from build123d import *

# Parameters (mm, degrees)
PAD_DEPTH       = 24
SKETCH_R        = 4.625
SKETCH_R_2      = 3
SKETCH_W        = 8.497862
SKETCH_H        = 16.9564
POCKET_DEPTH    = 4
SKETCH003_R     = 2.6
POCKET001_DEPTH = 13
FILLET_R        = 13
FILLET001_R     = 1
SKETCH004_R     = 3.2
POCKET002_DEPTH = 3


with BuildPart() as part:
    # Sketch002 → Pad (new body, symmetric)
    with BuildSketch(Plane.YZ.offset(24)):
        Polygon((0, 4), (56.5, 4), (56.5, -8), (48.5, -8), (48.5, -4), (52.5, -4), (52.5, 0), (13, 0), (13, -13), (0, -13), (0, 0), (-68, 0), (-68, 4), align=None)
    extrude(amount=PAD_DEPTH, both=True)

    # Sketch (on Face13 of Pad) → Pocket (cut)
    with BuildSketch(Plane(origin=(24, -34, 4), x_dir=(-1, 0, 0), z_dir=(0, 0, 1))):
        with Locations((-12.025, 28)):
            Circle(SKETCH_R)
        with Locations((12.025, 28)):
            Circle(SKETCH_R)
        with Locations((12.025, -28)):
            Circle(SKETCH_R)
        with Locations((-12.025, -28)):
            Circle(SKETCH_R)
        with Locations((-12.024955, 15.059916)):
            Circle(SKETCH_R_2)
        with Locations((12.024955, 15.059916)):
            Circle(SKETCH_R_2)
        with Locations((12.024955, -15.059916)):
            Circle(SKETCH_R_2)
        with Locations((-12.024955, -15.059916)):
            Circle(SKETCH_R_2)
        with Locations((-12.001069, 0.0218)):
            Rectangle(SKETCH_W, SKETCH_H)
        with Locations((12.001069, -0.0218)):
            Rectangle(SKETCH_W, SKETCH_H)
    extrude(amount=-POCKET_DEPTH, mode=Mode.SUBTRACT)

    # Sketch003 (on Face30 of Pocket) → Pocket001 (cut)
    with BuildSketch(Plane(origin=(24, 0, 0), x_dir=(0, 0, -1), z_dir=(0, -1, 0))):
        with Locations((9.313336, 0)):
            Circle(SKETCH003_R)
    extrude(amount=-POCKET001_DEPTH, mode=Mode.SUBTRACT)

    # Fillet
    fillet_edges = [part.edges().sort_by_distance(p)[0] for p in [
        (48, 6.5, -13),
        (0, 6.5, -13),
    ]]
    fillet(fillet_edges, radius=FILLET_R)

    # Fillet001
    fillet001_edges = [part.edges().sort_by_distance(p)[0] for p in [
        (24, 56.5, 4),
        (0, 56.5, -2),
        (48, 56.5, -2),
        (24, 56.5, -8),
        (0, 52.5, -8),
        (48, 52.5, -8),
        (24, 48.5, -8),
        (0, 6.5, 0),
        (0, 32.75, 0),
        (0, -34, 0),
        (0, 52.5, -2),
        (0, -68, 2),
        (0, 50.5, -4),
        (0, -34, 4),
        (0, 48.5, -6),
        (0, 28.25, 4),
        (48, 6.5, 0),
        (48, 32.75, 0),
        (48, -34, 0),
        (48, 52.5, -2),
        (48, -68, 2),
        (48, 50.5, -4),
        (48, -34, 4),
        (48, 48.5, -6),
        (48, 28.25, 4),
        (24, -68, 4),
        (24, -68, 0),
        (24, 48.5, -4),
    ]]
    fillet(fillet001_edges, radius=FILLET001_R)

    # Sketch004 (on Face5 of Fillet001) → Pocket002 (cut)
    with BuildSketch(Plane(origin=(24, 0, 0), x_dir=(0, 0, -1), z_dir=(0, -1, 0))):
        with Locations((9.313336, 0)):
            Circle(SKETCH004_R)
    extrude(amount=-POCKET002_DEPTH, mode=Mode.SUBTRACT)


solid = part.part
Read the model definition and answer for the solid it produces. Units are mm, in the model's axes. A direction names the side the tool comes from. Coordinates: 2 decimals unless noted, no trailing zeros. Loops run counter-clockwise (first coordinate to the right, second up) from the corner with the lowest first, then second, coordinate; pieces in that order, holes last. Notation, with made-up numbers: (-28.75, -8.75) - (8.25, -8.75) arc R16 cw to (8.25, 1.25) - close; hole circle Ø8 at (-20, 42.25). An arc over 180 degrees is marked (long way). Answer in a Markdown table with one row per item.
Q1. The mould has two halves that part along Y. Classify faces 1 (the flat face through (24, 56.5, -2)), 2 (the flat face through (48, 4, 1)), 3 (the cylindrical face through (7.7, -4.23, 2.03)): pulls with the +Y half, pulls with the -Y half, needs draft (parallel to the pull), parting line crosses it, or undercut.
Here are the results:
| item | result |
|---|---|
| face 1 | pulls with the +Y half |
| face 2 | needs draft |
| face 3 | undercut |
Q2. For faces 4 (the flat face through (24, 53, -8)), 5 (the flat face through (7.75, -34, 2)), 6 (the flat face through (24, 51, -4)), determine the directions among +Z, -Z, +X, -X, +Y, -Y from which every point of the face is accessible in a straight line to the end or side of a thin tool.
Here are the results:
| item | result |
|---|---|
| face 4 | -Z, +X, -X, +Y |
| face 5 | +Z, -Z |
| face 6 | +X, -X |
Q3. Find section B-B on x = 24. Write down the section's boundary in (y, z), plus the area to 3 significant figures.
Here are the results:
| item | result |
|---|---|
| outline | (-68, 1) arc R1 ccw to (-67, 0) - (0, 0) - (0, -6.11) - (3, -6.11) - (3, -6.71) - (13, -6.71) - (13, 0) - (52.5, 0) - (52.5, -4) - (49.5, -4) arc R1 ccw to (48.5, -5) - (48.5, -7) arc R1 ccw to (49.5, -8) - (55.5, -8) arc R1 ccw to (56.5, -7) - (56.5, 3) arc R1 ccw to (55.5, 4) - (-67, 4) arc R1 ccw to (-68, 3) - close; (0, -13) - (13, -13) - (13, -11.91) - (3, -11.91) - (3, -12.51) - (0, -12.51) - close |
| area | 643 mm^2 |
Q4. Straight lines are drawn through the part: line 1 along X through (y, z) = (-6, 2.7); line 2 along Y through (x, z) = (20.5, -0.5); line 3 along Y through (x, z) = (25, -6.5). For each, find the intervals that lie inside material, in ascending order. Write a range as [from, to].
Here are the results:
| item | result |
|---|---|
| line 1 | x = [0, 7.35], [16.6, 31.4], [40.65, 48] |
| line 2 | y = [0, 13], [52.5, 56.5] |
| line 3 | y = [3, 13], [48.5, 56.5] |
Q5. Find section A-A on y = -30. Write down the section's boundary in (x, z), plus the area to 3 significant figures.
Here are the results:
| item | result |
|---|---|
| outline | (0, 1) arc R1 ccw to (1, 0) - (7.75, 0) - (7.75, 4) - (1, 4) arc R1 ccw to (0, 3) - close; (16.25, 0) - (31.75, 0) - (31.75, 4) - (16.25, 4) - close; (40.25, 0) - (47, 0) arc R1 ccw to (48, 1) - (48, 3) arc R1 ccw to (47, 4) - (40.25, 4) - close |
| area | 123 mm^2 |
Q6. Given P1, Ø10, axis at y = -15.5, z = -4.5, coming from the -X side; P2, Ø2, axis at x = 14, z = -1.5, coming from the -Y side; P3, Ø6, axis at x = 24, z = -9.31, coming from the -Y side, each flat-ended and moving along its own axis, determine where each tip first touches the part or whether it passes through.
Here are the results:
| item | result |
|---|---|
| P1 | stops at x = 0.13 |
| P2 | stops at y = 0 |
| P3 | stops at y = 3 |
Q7. Find section D-D on y = -12. Write down the section's boundary in (x, z), plus the area to 3 significant figures.
Here are the results:
| item | result |
|---|---|
| outline | (0, 1) arc R1 ccw to (1, 0) - (47, 0) arc R1 ccw to (48, 1) - (48, 3) arc R1 ccw to (47, 4) - (1, 4) arc R1 ccw to (0, 3) - close |
| area | 191 mm^2 |
Q8. Find section C-C on z = -2. Write down the section's boundary in (x, y).
Here are the results:
| item | result |
|---|---|
| outline | (0, 53.5) arc R1 ccw to (1, 52.5) - (47, 52.5) arc R1 ccw to (48, 53.5) - (48, 55.5) arc R1 ccw to (47, 56.5) - (1, 56.5) arc R1 ccw to (0, 55.5) - close; (0.15, 0) - (47.85, 0) - (47.85, 13) - (0.15, 13) - close |
